Autodesk Inventor part; units mm, degrees
ref_plane "YZ Plane" through (0, 0, 0) normal (1, 0, 0) x (0, 1, 0)
ref_plane "XZ Plane" through (0, 0, 0) normal (0, 1, 0) x (-1, 0, 0)
ref_plane "XY Plane" through (0, 0, 0) normal (0, 0, 1) x (1, 0, 0)
sketch "Sketch1" plane through (0, 0, 0) normal (0, 0, 1) x (1, 0, 0)
  line L0 (0, 201.6) -> (0, -201.6) construction
  circle A0 centre (17.361, 111.95) radius 2 construction
  circle A1 centre (17.361, 85.95) radius 2 construction
  circle A2 centre (17.361, 59.95) radius 2 construction
  circle A3 centre (17.361, 33.95) radius 2 construction
  circle A4 centre (17.361, 7.95) radius 2 construction
  circle A5 centre (17.361, -25.35) radius 2 construction
  circle A6 centre (17.361, -51.35) radius 2 construction
  circle A7 centre (17.361, -77.35) radius 2 construction
  circle A8 centre (17.361, -103.35) radius 2 construction
  circle A9 centre (17.361, -129.35) radius 2 construction
  circle A10 centre (17.361, -116.35) radius 2 construction
  circle A11 centre (17.361, -90.35) radius 2 construction
  circle A12 centre (17.361, -64.35) radius 2 construction
  circle A13 centre (17.361, -38.35) radius 2 construction
  circle A14 centre (17.361, -12.35) radius 2 construction
  circle A15 centre (17.361, 20.95) radius 2 construction
  circle A16 centre (17.361, 46.95) radius 2 construction
  circle A17 centre (17.361, 72.95) radius 2 construction
  circle A18 centre (17.361, 98.95) radius 2 construction
  circle A19 centre (17.361, 124.95) radius 2 construction
  circle A20 centre (8, -12) radius 2.65 construction
  circle A21 centre (8, -52) radius 2.65 construction
  circle A22 centre (8, -92) radius 2.65 construction
  circle A23 centre (8, -132) radius 2.65 construction
  circle A24 centre (34, -112) radius 2.65 construction
  circle A25 centre (34, -72) radius 2.65 construction
  circle A26 centre (34, -32) radius 2.65 construction
  circle A27 centre (34, 8) radius 2.65 construction
  circle A28 centre (34, 48) radius 2.65 construction
  circle A29 centre (8, 28) radius 2.65 construction
  circle A30 centre (8, 68) radius 2.65 construction
  circle A31 centre (8, 88) radius 2.65 construction
  circle A32 centre (8, 108) radius 2.65 construction
  circle A33 centre (8, 128) radius 2.65 construction
  circle A34 centre (68, 118) radius 2.65 construction
  circle A35 centre (55, 95.7) radius 2.65 construction
  circle A36 centre (55, 69.7) radius 2.65 construction
  circle A37 centre (55, 43.7) radius 2.65 construction
  circle A38 centre (55, 17.7) radius 2.65 construction
  circle A39 centre (55, -2.3) radius 2.65 construction
  circle A40 centre (55, -28.3) radius 2.65 construction
  circle A41 centre (55, -54.3) radius 2.65 construction
  circle A42 centre (55, -80.3) radius 2.65 construction
  circle A43 centre (55, -106.3) radius 2.65 construction
  circle A44 centre (55, -132.3) radius 2.65 construction
  circle A45 centre (68, -136) radius 2.65 construction
  circle A46 centre (68, -110) radius 2.65 construction
  circle A47 centre (68, -84) radius 2.65 construction
  circle A48 centre (68, -58) radius 2.65 construction
  circle A49 centre (68, -32) radius 2.65 construction
  circle A50 centre (68, -6) radius 2.65 construction
  circle A51 centre (68, 14) radius 2.65 construction
  circle A52 centre (68, 40) radius 2.65 construction
  circle A53 centre (68, 66) radius 2.65 construction
  circle A54 centre (68, 92) radius 2.65 construction
  circle A55 centre (55, 121.7) radius 2.65 construction
  circle A56 centre (34, 128) radius 2.65 construction
  circle A57 centre (34, 108) radius 2.65 construction
  circle A58 centre (34, 88) radius 2.65 construction
  circle A59 centre (8, 48) radius 2.65 construction
  circle A60 centre (34, 68) radius 2.65 construction
  circle A61 centre (34, 28) radius 2.65 construction
  circle A62 centre (34, -12) radius 2.65 construction
  circle A63 centre (34, -52) radius 2.65 construction
  circle A64 centre (34, -92) radius 2.65 construction
  circle A65 centre (34, -132) radius 2.65 construction
  circle A66 centre (8, -112) radius 2.65 construction
  circle A67 centre (8, -72) radius 2.65 construction
  circle A68 centre (8, -32) radius 2.65 construction
  circle A69 centre (8, 8) radius 2.65 construction
  line L1 (75, 142) -> (75, -142)
  line L2 (0, 142) -> (75, 142)
  line L3 (0, -142) -> (0, 142)
  line L4 (75, -142) -> (0, -142) construction
  line L5 (-2, -144) -> (-2, 144)
  line L6 (-2, 144) -> (77, 144)
  line L7 (77, 144) -> (77, -144)
  line L8 (77, -144) -> (-2, -144)
  circle A70 centre (8, -132) radius 2.05
  circle A71 centre (8, -112) radius 2.05
  circle A72 centre (8, -92) radius 2.05
  circle A73 centre (8, -72) radius 2.05
  circle A74 centre (8, -52) radius 2.05
  circle A75 centre (8, -32) radius 2.05
  circle A76 centre (8, -12) radius 2.05
  circle A77 centre (8, 8) radius 2.05
  circle A78 centre (8, 28) radius 2.05
  circle A79 centre (8, 48) radius 2.05
  circle A80 centre (8, 68) radius 2.05
  circle A81 centre (8, 88) radius 2.05
  circle A82 centre (8, 108) radius 2.05
  circle A83 centre (8, 128) radius 2.05
  circle A84 centre (17.361, 124.95) radius 1.55
  circle A85 centre (17.361, 111.95) radius 1.55
  circle A86 centre (17.361, 98.95) radius 1.55
  circle A87 centre (17.361, 85.95) radius 1.55
  circle A88 centre (17.361, 72.95) radius 1.55
  circle A89 centre (17.361, 59.95) radius 1.55
  circle A90 centre (17.361, 46.95) radius 1.55
  circle A91 centre (17.361, 33.95) radius 1.55
  circle A92 centre (17.361, 20.95) radius 1.55
  circle A93 centre (17.361, 7.95) radius 1.55
  circle A94 centre (17.361, -12.35) radius 1.55
  circle A95 centre (17.361, -25.35) radius 1.55
  circle A96 centre (17.361, -38.35) radius 1.55
  circle A97 centre (17.361, -51.35) radius 1.55
  circle A98 centre (17.361, -64.35) radius 1.55
  circle A99 centre (17.361, -77.35) radius 1.55
  circle A100 centre (17.361, -90.35) radius 1.55
  circle A101 centre (17.361, -103.35) radius 1.55
  circle A102 centre (17.361, -116.35) radius 1.55
  circle A103 centre (17.361, -129.35) radius 1.55
  circle A104 centre (34, -132) radius 2.05
  circle A105 centre (34, -112) radius 2.05
  circle A106 centre (34, -92) radius 2.05
  circle A107 centre (34, -72) radius 2.05
  circle A108 centre (34, -52) radius 2.05
  circle A109 centre (34, -32) radius 2.05
  circle A110 centre (34, -12) radius 2.05
  circle A111 centre (34, 8) radius 2.05
  circle A112 centre (34, 28) radius 2.05
  circle A113 centre (34, 48) radius 2.05
  circle A114 centre (34, 68) radius 2.05
  circle A115 centre (34, 88) radius 2.05
  circle A116 centre (34, 108) radius 2.05
  circle A117 centre (34, 128) radius 2.05
  circle A118 centre (55, 121.7) radius 2.05
  circle A119 centre (68, 118) radius 2.05
  circle A120 centre (55, 95.7) radius 2.05
  circle A121 centre (68, 92) radius 2.05
  circle A122 centre (55, 69.7) radius 2.05
  circle A123 centre (68, 66) radius 2.05
  circle A124 centre (55, 43.7) radius 2.05
  circle A125 centre (55, 17.7) radius 2.05
  circle A126 centre (68, 40) radius 2.05
  circle A127 centre (68, 14) radius 2.05
  circle A128 centre (55, -2.3) radius 2.05
  circle A129 centre (68, -6) radius 2.05
  circle A130 centre (55, -28.3) radius 2.05
  circle A131 centre (68, -32) radius 2.05
  circle A132 centre (55, -54.3) radius 2.05
  circle A133 centre (68, -58) radius 2.05
  circle A134 centre (55, -80.3) radius 2.05
  circle A135 centre (55, -106.3) radius 2.05
  circle A136 centre (68, -84) radius 2.05
  circle A137 centre (68, -110) radius 2.05
  circle A138 centre (55, -132.3) radius 2.05
  circle A139 centre (68, -136) radius 2.05
  dimension "d10" = 2
  dimension "d11" = 4.1
  dimension "d12" = 3.1
extrude "Extrusion4" add sketch "Sketch1" along normal blind 0.2
properties part number "17-0028-0027"
Input: part model. Units: mm. Frame: model coordinates. Give positions to 0.01 mm unless a question says otherwise; leave off trailing zeros.
1. Material intervals for L1, parallel to X at y = -132.3, z = 0.15; L2, parallel to X at y = 64.5, z = 0.1; L3, parallel to X at y = 92.5, z = 0.1, sorted ascending.
Derived:
L1: x = -2 to 5.97, 10.03 to 31.97, 36.03 to 52.95, 57.05 to 77
L2: x = -2 to 66.6, 69.4 to 77
L3: x = -2 to 66.01, 69.99 to 77
2. Pin query (flat end, axial travel): pin 1 (4.5 mm diameter, centred on x = 8, y = -12, fed in from -Z). Return the tip coordinate at first contact, or that it passes through.
Derived:
pin 1: stops at z = 0
3. Section A-A on z = 0.15. Give the number of separate pieces and of enclosed holes in the cut face, and give its area (3 significant figures).
Derived:
separate pieces: 1
enclosed holes: 70
area: 21,900 mm2
